from build123d import *

# Parameters (mm, degrees)
BOX001_W                    = 180
BOX001_H                    = 180
BOX001_DEPTH                = 2
BOX_W                       = 180
BOX_H                       = 180
BOX_DEPTH                   = 1
CYLINDER494_R               = 1.5
CYLINDER494_DEPTH           = 60
CYLINDER494_PLACEMENT_ANGLE = 45
CYLINDER495_R               = 1.5
CYLINDER495_DEPTH           = 60
CYLINDER496_R               = 1.5
CYLINDER496_DEPTH           = 60
CYLINDER496_PLACEMENT_ANGLE = 135
CYLINDER498_R               = 1.5
CYLINDER498_DEPTH           = 60
CYLINDER498_PLACEMENT_ANGLE = 225
CYLINDER499_R               = 1.5
CYLINDER499_DEPTH           = 60
CYLINDER500_R               = 1.5
CYLINDER500_DEPTH           = 60
CYLINDER500_PLACEMENT_ANGLE = 45
CYLINDER_R                  = 1.5
CYLINDER_DEPTH              = 60
TUBE029_R                   = 74
TUBE029_R_2                 = 61
TUBE029_DEPTH               = 2


with BuildPart() as krychle001:
    # Box001 → Box001 (new body)
    with BuildSketch(Plane(origin=(-90, -186, 14), x_dir=(1, 0, 0), z_dir=(0, 0, 1))):
        with Locations((90, 90)):
            Rectangle(BOX001_W, BOX001_H)
    extrude(amount=BOX001_DEPTH)


with BuildPart() as krychle:
    # Box → Box (new body)
    with BuildSketch(Plane(origin=(-90, -174, 14), x_dir=(1, 0, 0), z_dir=(0, 0, 1))):
        with Locations((90, 90)):
            Rectangle(BOX_W, BOX_H)
    extrude(amount=BOX_DEPTH)


with BuildPart() as obj1:
    # Cylinder494 → Cylinder494 (new body)
    with BuildSketch(Plane.XY):
        Circle(CYLINDER494_R)
    extrude(amount=CYLINDER494_DEPTH)


with BuildPart() as obj1_1:
    # Cylinder494 placement: moved
    add(obj1.part.moved(Location((50.204581, -50.204581, 0))).rotate(Axis((50.204581, -50.204581, 0), (0, 0, 1)), CYLINDER494_PLACEMENT_ANGLE))


with BuildPart() as obj2:
    # Cylinder495 → Cylinder495 (new body)
    with BuildSketch(Plane(origin=(71, 0, 0), x_dir=(0, 1, 0), z_dir=(0, 0, 1))):
        Circle(CYLINDER495_R)
    extrude(amount=CYLINDER495_DEPTH)


with BuildPart() as obj3:
    # Cylinder496 → Cylinder496 (new body)
    with BuildSketch(Plane.XY):
        Circle(CYLINDER496_R)
    extrude(amount=CYLINDER496_DEPTH)


with BuildPart() as obj3_1:
    # Cylinder496 placement: moved
    add(obj3.part.moved(Location((50.204581, 50.204581, 0))).rotate(Axis((50.204581, 50.204581, 0), (0, 0, 1)), CYLINDER496_PLACEMENT_ANGLE))


with BuildPart() as obj4:
    # Cylinder498 → Cylinder498 (new body)
    with BuildSketch(Plane.XY):
        Circle(CYLINDER498_R)
    extrude(amount=CYLINDER498_DEPTH)


with BuildPart() as obj4_1:
    # Cylinder498 placement: moved
    add(obj4.part.moved(Location((-50.204581, 50.204581, 0))).rotate(Axis((-50.204581, 50.204581, 0), (0, 0, 1)), CYLINDER498_PLACEMENT_ANGLE))


with BuildPart() as obj5:
    # Cylinder499 → Cylinder499 (new body)
    with BuildSketch(Plane(origin=(-71, 0, 0), x_dir=(0, -1, 0), z_dir=(0, 0, 1))):
        Circle(CYLINDER499_R)
    extrude(amount=CYLINDER499_DEPTH)


with BuildPart() as obj6:
    # Cylinder500 → Cylinder500 (new body)
    with BuildSketch(Plane.XY):
        Circle(CYLINDER500_R)
    extrude(amount=CYLINDER500_DEPTH)


with BuildPart() as obj6_1:
    # Cylinder500 placement: moved
    add(obj6.part.moved(Location((-50.204581, -50.204581, 0))).rotate(Axis((-50.204581, -50.204581, 0), (0, 0, -1)), CYLINDER500_PLACEMENT_ANGLE))


with BuildPart() as compound330:
    # Cylinder → Cylinder (new body)
    with BuildSketch(Plane(origin=(0, -71, 0), x_dir=(1, 0, 0), z_dir=(0, 0, 1))):
        Circle(CYLINDER_R)
    extrude(amount=CYLINDER_DEPTH)

    # Compound330: union obj1, obj2, obj3, obj4, obj5, obj6
    add(obj1_1.part)
    add(obj2.part)
    add(obj3_1.part)
    add(obj4_1.part)
    add(obj5.part)
    add(obj6_1.part)


with BuildPart() as obj7:
    # Tube029 → Tube029 (new body)
    with BuildSketch(Plane.XY.offset(14)):
        Circle(TUBE029_R)
        Circle(TUBE029_R_2, mode=Mode.SUBTRACT)
    extrude(amount=TUBE029_DEPTH)

    # Cut204: cut Compound330
    add(compound330.part, mode=Mode.SUBTRACT)

    # Cut: cut Krychle
    add(krychle.part, mode=Mode.SUBTRACT)

    # Cut206: cut Krychle001
    add(krychle001.part, mode=Mode.SUBTRACT)


solid = obj7.part
For this review, take the finished solid that the model builds, in its own axes (mm). A direction names the side the tool comes from. Give positions to 0.01 mm unless a question says otherwise; leave off trailing zeros. Order: outer loops, then holes, each group sorted by start corner. A loop starts at its lowest first (then second) coordinate and runs counter-clockwise, first axis right, second up. Notation, with made-up numbers: (41, -8) - (67, -8) arc R8 ccw to (67, 4) - close; hole circle Ø11 at (4, 33.25). An arc over 180 degrees is marked (long way). Answer as a JSON object with one key per item and string values. Group by question number.
Item 1: Take a section at D-D on x = 0. Give the boundary of the cut face in (y, z).
Item 2: Take a section at C-C on y = 22. Give the boundary of the cut face in (x, z), and give its area (3 significant figures).
Item 3: Take a section at B-B on x = -71. Give the boundary of the cut face in (y, z), and give its area (3 significant figures).
Item 4: Take a section at A-A on y = 0. Give the boundary of the cut face in (x, z).
Item 5: Machinability: for faces 4 (the cylindrical face through (49.291, 49.015, 14.986)), 5 (the flat face through (-67, 0, 15)), which of the approach directions +Z, -Z, +X, -X, +Y, -Y give a long, thin tool a straight path to every point of the face, cutting with its end or side? Answer none if there is none.
Item 6: Draft analysis for pull direction Y (two halves, no side actions). For faces 1 (the cylindrical face through (-69.735, -0.806, 15.493)), 2 (the flat face through (67, 0, 15)), 3 (the cylindrical face through (69.735, 0.806, 15.493)), state which applies: pulls with the +Y half, pulls with the -Y half, needs draft (parallel to the pull), parting line crosses it, or undercut.
Item 7: Clearance check with a flat-ended pin moving along its axis: pin 1 Ø3.5 at (x, y) = (-65.5, -0.5) entering from -Z. State where the tip first meets the part, or that it passes through.
Item 8: Wall thickness on line 1 along X through (y, z) = (0, 15.65); line 2 along X through (y, z) = (50, 15.75); line 3 along Y through (x, z) = (0, 15.15): over which ranges is each line inside the solid? List them lowest first.
Reported:
{
 "1": {"outline": "(61, 14) - (74, 14) - (74, 16) - (61, 16) - close"},
 "2": {"outline": "(-70.65, 14) - (-56.89, 14) - (-56.89, 16) - (-70.65, 16) - close; (56.89, 14) - (70.65, 14) - (70.65, 16) - (56.89, 16) - close", "area": "55.0 mm^2"},
 "3": {"outline": "(-6, 15) - (-1.5, 15) - (-1.5, 16) - (-6, 16) - close; (1.5, 15) - (6, 15) - (6, 14) - (20.86, 14) - (20.86, 16) - (1.5, 16) - close", "area": "38.7 mm^2"},
 "4": {"outline": "(-74, 15) - (-72.5, 15) - (-72.5, 16) - (-74, 16) - close; (-69.5, 15) - (-61, 15) - (-61, 16) - (-69.5, 16) - close; (61, 15) - (69.5, 15) - (69.5, 16) - (61, 16) - close; (72.5, 15) - (74, 15) - (74, 16) - (72.5, 16) - close"},
 "5": {"face 4": "+Z, -Z", "face 5": "-Z, +X, -X, -Y"},
 "6": {"face 1": "undercut", "face 2": "needs draft", "face 3": "undercut"},
 "7": {"pin 1": "z = 15"},
 "8": {"line 1": "-74 to -72.5, -69.5 to -61, 61 to 69.5, 72.5 to 74", "line 2": "-54.55 to -51.69, -48.72 to -34.94, 34.94 to 48.72, 51.69 to 54.55", "line 3": "61 to 74"}
}
